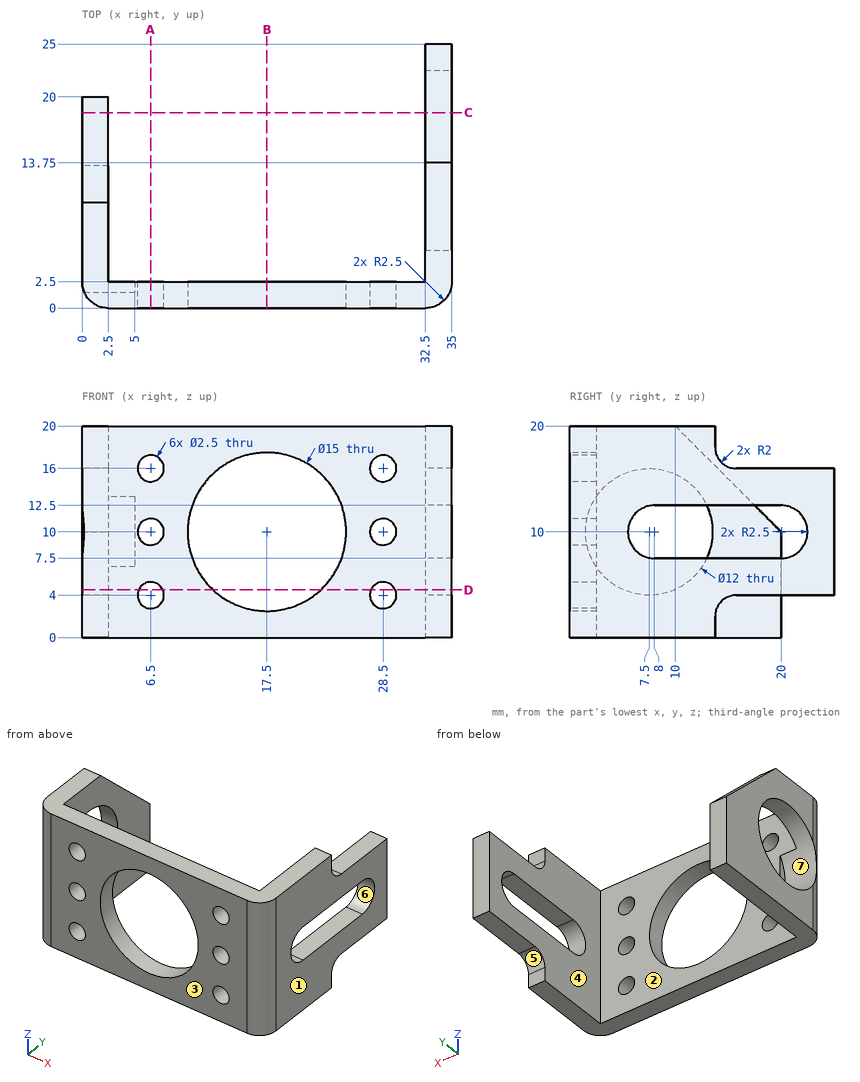
Input: dimensioned drawing with shaded views. Units: mm. Origin: part minimum x, y, z. A direction names the side the tool comes from. Coordinates: 2 decimals unless noted, no trailing zeros. Loops run counter-clockwise (first coordinate to the right, second up) from the corner with the lowest first, then second, coordinate; pieces in that order, holes last.
Q1. Section B-B, the plane x = 17.5. Return the cut outline in (y, z), and give its area (3 significant figures).
Results are:
outline: (0, 0) - (2.5, 0) - (2.5, 2.5) - (0, 2.5) - close; (0, 17.5) - (2.5, 17.5) - (2.5, 20) - (0, 20) - close
area: 12.5 mm2
Q2. Section D-D, the plane z = 4.5. Return the cut outline in (x, y), and give its area (3 significant figures).
Results are:
outline: (0, 2.5) arc R2.5 ccw to (2.5, 0) - (5.35, 0) - (5.35, 2.5) - (2.5, 2.5) - (2.5, 5.1) - (0, 5.1) - close; (0, 9.9) - (2.5, 9.9) - (2.5, 20) - (0, 20) - close; (7.65, 0) - (12.4, 0) - (12.4, 2.5) - (7.65, 2.5) - close; (22.6, 0) - (27.35, 0) - (27.35, 2.5) - (22.6, 2.5) - close; (29.65, 0) - (32.5, 0) arc R2.5 ccw to (35, 2.5) - (35, 25) - (32.5, 25) - (32.5, 2.5) - (29.65, 2.5) - close
area: 136 mm2
Q3. Set-up query: the marked faces 4, 5, 6 and 7. Return all of +Z, -Z, +X, -X, +Y, -Y with unobstructed straight access to the full face (end or side cutting, diameter ignored); none if empty.
Results are:
face 4: +Z, -Z, +Y
face 5: -Z, +X, +Y
face 6: +X, -X
face 7: -X
Q4. Line query: line 1 along Z through (x, y) = (28.5, 0.9); line 2 along Y through (x, z) = (12.5, 2.5); line 3 along X through (y, z) = (3.75, 17.5). Output: solid intervals per line, ascending.
Results are:
line 1: z = 0 to 2.75, 5.25 to 8.75, 11.25 to 14.75, 17.25 to 20
line 2: y = 0 to 2.5
line 3: x = 0 to 2.5, 32.5 to 35
Q5. Section C-C, the plane y = 18.5. Return the cut outline in (x, z).
Results are:
outline: (0, 0) - (2.5, 0) - (2.5, 11.5) - (0, 11.5) - close; (32.5, 4) - (35, 4) - (35, 7.5) - (32.5, 7.5) - close; (32.5, 12.5) - (35, 12.5) - (35, 16) - (32.5, 16) - close
Q6. Section A-A, the plane x = 6.5. Return the cut outline in (y, z), and give its area (4 significant figures).
Results are:
outline: (0, 0) - (2.5, 0) - (2.5, 2.75) - (0, 2.75) - close; (0, 5.25) - (2.5, 5.25) - (2.5, 8.75) - (0, 8.75) - close; (0, 11.25) - (2.5, 11.25) - (2.5, 14.75) - (0, 14.75) - close; (0, 17.25) - (2.5, 17.25) - (2.5, 20) - (0, 20) - close
area: 31.25 mm2
Q7. Contact query for flat-ended pins moving along their axis: pin 1 (5 mm diameter, centred on x = 7, z = 17, fed in from +Y); pin 2 (0.5 mm diameter, centred on y = 2, z = 10.5, fed in from -X); pin 3 (2 mm diameter, centred on x = 6.5, z = 10, fed in from +Y); pin 4 (12 mm diameter, centred on x = 6.5, z = 10, fed in from +Y). Output: stop coordinate, or through.
Results are:
pin 1: stops at y = 2.5
pin 2: stops at x = 5
pin 3: passes through
pin 4: stops at y = 20
Q8. Mould query, pull axis X, two halves, no side actions, for the marked faces 1, 2 and 3. Classes: +X half, -X half, draft (parallel to the pull), parting line (faces both ways), or undercut.
Results are:
face 1: +X half
face 2: undercut
face 3: draft
